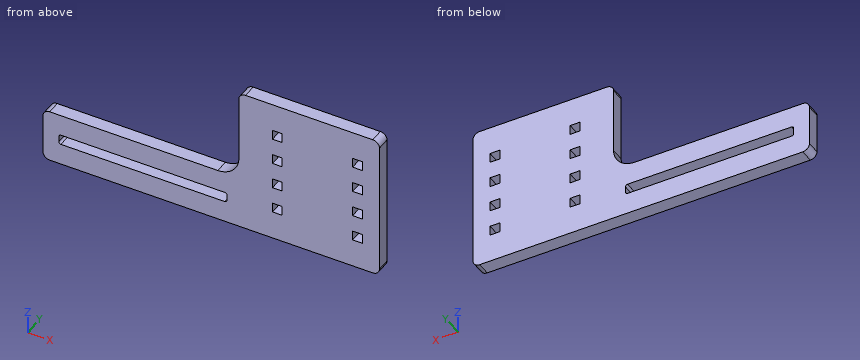
```python
from build123d import *

# Parameters (mm, degrees)
SKETCH1_W           = 80
SKETCH1_H           = 4.819787269
SKETCH1_W_2         = 4.6228
SKETCH1_H_2         = 4.6228
BOSS_EXTRUDE1_DEPTH = 6.35
FILLET2_R           = 3.175
FILLET3_R           = 3.175
FILLET4_R           = 10
FILLET5_R           = 1


with BuildPart() as part:
    # Sketch1 → Boss-Extrude1 (new body)
    with BuildSketch(Plane(origin=(0, 0, 0), x_dir=(1, 0, 0), z_dir=(0, 1, 0))):
        Polygon((0, 0), (160, 0), (160, -70), (93.1472, -70), (93.1472, -25.4), (0, -25.4), align=None)
        with Locations((47.5, -12.740106366)):
            Rectangle(SKETCH1_W, SKETCH1_H, mode=Mode.SUBTRACT)
        with Locations((149.5586, -15.96068286)):
            Rectangle(SKETCH1_W_2, SKETCH1_H_2, mode=Mode.SUBTRACT)
        with Locations((149.5586, -28.71348286)):
            Rectangle(SKETCH1_W_2, SKETCH1_H_2, mode=Mode.SUBTRACT)
        with Locations((149.5586, -41.46628286)):
            Rectangle(SKETCH1_W_2, SKETCH1_H_2, mode=Mode.SUBTRACT)
        with Locations((111.4586, -15.96068286)):
            Rectangle(SKETCH1_W_2, SKETCH1_H_2, mode=Mode.SUBTRACT)
        with Locations((111.4586, -28.71348286)):
            Rectangle(SKETCH1_W_2, SKETCH1_H_2, mode=Mode.SUBTRACT)
        with Locations((111.4586, -41.46628286)):
            Rectangle(SKETCH1_W_2, SKETCH1_H_2, mode=Mode.SUBTRACT)
        with Locations((149.5586, -54.21908286)):
            Rectangle(SKETCH1_W_2, SKETCH1_H_2, mode=Mode.SUBTRACT)
        with Locations((111.4586, -54.21908286)):
            Rectangle(SKETCH1_W_2, SKETCH1_H_2, mode=Mode.SUBTRACT)
    extrude(amount=BOSS_EXTRUDE1_DEPTH)

    # Fillet2
    fillet2_edges = [part.edges().sort_by_distance(p)[0] for p in [
        (0, 3.175, 25.4),
    ]]
    fillet(fillet2_edges, radius=FILLET2_R)

    # Fillet3
    fillet3_edges = [part.edges().sort_by_distance(p)[0] for p in [
        (0, 3.175, 0),
        (160, 3.175, 0),
        (160, 3.175, 70),
        (93.1472, 3.175, 70),
    ]]
    fillet(fillet3_edges, radius=FILLET3_R)

    # Fillet4
    fillet4_edges = [part.edges().sort_by_distance(p)[0] for p in [
        (93.1472, 3.175, 25.4),
    ]]
    fillet(fillet4_edges, radius=FILLET4_R)

    # Fillet5
    fillet5_edges = [part.edges().sort_by_distance(p)[0] for p in [
        (7.5, 3.175, 10.330212731),
        (7.5, 3.175, 15.15),
        (87.5, 3.175, 15.15),
        (87.5, 3.175, 10.330212731),
    ]]
    fillet(fillet5_edges, radius=FILLET5_R)


solid = part.part
```
Work out the finished part from the listing and answer in its coordinate system (mm). Give positions to 0.01 mm unless a question says otherwise; leave off trailing zeros. Order: outer loops, then holes, each group sorted by start corner. A loop starts at its lowest first (then second) coordinate and runs counter-clockwise, first axis right, second up. Notation, with made-up numbers: M 65,-20 L 115,-20 A11 cw 115,1 Z; hole C -2,-31 d6. An arc over 180 degrees is marked long. Return JSON: item names as keys, results as strings.
1) Section B-B, the plane y = 4.5 is taken. Give the number of separate pieces and of enclosed holes in the cut face, plus the area to 3 significant figures.
Resolved:
{"separate pieces": "1", "enclosed holes": "9", "area": "6,500 mm^2"}
2) Section D-D, the plane z = 34 is taken. Write down the section's boundary in (x, y), plus the area to 3 significant figures.
Resolved:
{"outline": "M 93.05,0 L 160,0 L 160,6.35 L 93.05,6.35 Z", "area": "425 mm^2"}
3) Straight lines are drawn through the part: line 1 along Z through (x, y) = (113.5, 2.75); line 2 along X through (y, z) = (1.25, 42); line 3 along Z through (x, y) = (27, 4.75). For each, find the intervals that lie inside material, in ascending order. Write a range as [from, to].
Resolved:
{"line 1": "[0, 13.65], [18.27, 26.4], [31.02, 39.15], [43.78, 51.91], [56.53, 70]", "line 2": "[93.15, 109.15], [113.77, 147.25], [151.87, 160]", "line 3": "[0, 10.33], [15.15, 25.4]"}
4) Section C-C, the plane z = 48 is taken. Write down the section's boundary in (x, y).
Resolved:
{"outline": "M 93.15,0 L 160,0 L 160,6.35 L 93.15,6.35 Z"}
5) Section A-A, the plane x = 63 is taken. Write down the section's boundary in (y, z), plus the area to 3 significant figures.
Resolved:
{"outline": "M 0,0 L 6.35,0 L 6.35,10.33 L 0,10.33 Z; M 0,15.15 L 6.35,15.15 L 6.35,25.4 L 0,25.4 Z", "area": "131 mm^2"}
6) Each of these flat-tipped pins is pushed along its axis until it touches: pin 1 (1.9 mm diameter, centred on x = 46.5, y = 3, fed in from +Z); pin 2 (3.5 mm diameter, centred on y = 2, z = 42, fed in from -X). Where does it stop, or does it pass through?
Resolved:
{"pin 1": "z = 25.4", "pin 2": "x = 93.15"}
